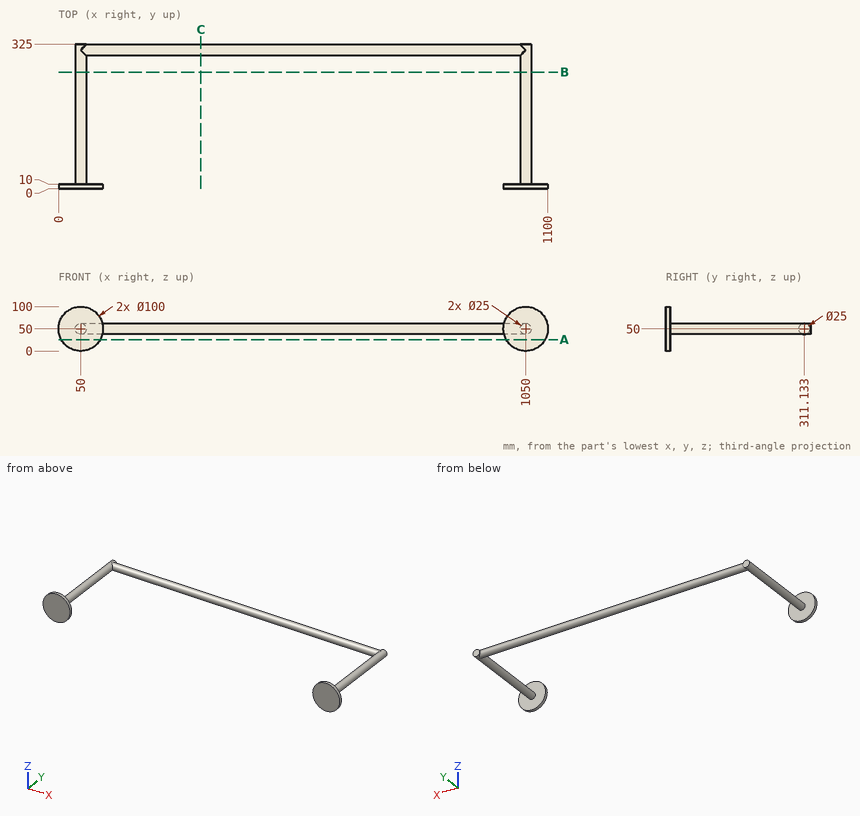
Study the drawing (mm; zero at the part's minimum x, y, z) and answer. Coordinates: 2 decimals unless noted, no trailing zeros. Loops run counter-clockwise (first coordinate to the right, second up) from the corner with the lowest first, then second, coordinate; pieces in that order, holes last. Notation, with made-up numbers: (43, 25) -> (85, 25) arc R14 cw to (85, 37) -> close; hole circle Ø8 at (84.25, -15). An arc over 180 degrees is marked (long way). Answer in a Markdown table with one row per item. Add a question column.
1. The part is cut by section B-B, the plane y = 262. Write down the section's boundary in (x, z), then the cut area to 3 significant figures.
2. The part is cut by section C-C, the plane x = 320. Write down the section's boundary in (y, z).
3. A flat-ended cylindrical pin translates along its axis: P1, Ø5, axis at y = 112, z = 43.5, coming from the +X side. Find the tip coordinate at first contact, or state that the pin passes through.
4. Consider line 1 (X direction, y = 154, z = 51); line 2 (Y direction, x = 431.5, z = 49); line 3 (Z direction, x = 558.5, y = 312). Determine where each line is inside the solid, lowest interval first. Write a range as [from, to].
5. The part is cut by section A-A, the plane z = 25.5. Write down the section's boundary in (x, y).
Answer below:
| question | item | result |
|---|---|---|
| 1 | outline | circle Ø25 at (50, 50); circle Ø25 at (1050, 50) |
| 1 | area | 982 mm2 |
| 2 | outline | circle Ø25 at (311.13, 50) |
| 3 | P1 | x = 1061.84 |
| 4 | line 1 | [37.54, 62.46], [1037.54, 1062.46] |
| 4 | line 2 | [298.67, 323.59] |
| 4 | line 3 | [37.53, 62.47] |
| 5 | outline | (6.41, 0) -> (93.59, 0) -> (93.59, 10) -> (6.41, 10) -> close; (1006.41, 0) -> (1093.59, 0) -> (1093.59, 10) -> (1006.41, 10) -> close |
